Here's how the part is built. I have some questions about the finished solid (model axes, mm). A direction names the side the tool comes from. Round coordinates to 2 decimals unless told otherwise and drop trailing zeros. Loops run counter-clockwise (first coordinate to the right, second up) from the corner with the lowest first, then second, coordinate; pieces in that order, holes last. Notation, with made-up numbers: (63, 84) - (92, 84) arc R22 cw to (92, 101) - close; hole circle Ø4 at (-20, 36). An arc over 180 degrees is marked (long way). Answer as a JSON object with one key per item and string values. Group by question number.
1) I want a section at B-B, the plane z = 1.75. Give the number of separate pieces and of enclosed holes in the cut face, then the cut area to 3 significant figures.
2) I want a section at A-A, the plane y = 2. Please give me the cut outline in (x, z).
3) If we mould it in two halves opening along X, with no side actions, what happens to faces 1 (the face through (29.626, 11.272, 3.904)), 2 (the face through (6.35, 12.19, 2.4))? For each: pulls with the +X half, pulls with the -X half, needs draft (parallel to the pull), parting line crosses it, or undercut.
4) If I drill on line 1 along X through (y, z) = (25.4, 2.25); line 2 along X through (y, z) = (13, 2.05); line 3 along Y through (x, z) = (24.8, 2.7), over which ranges is the centre line in solid material (lowest first)? Write a range as [from, to].
5) I want a section at C-C, the plane x = 9. Please give me the cut outline in (y, z), then the cut area to 3 significant figures.
6) Will these pins go through, and if not, where does the flat tip stop? P1, Ø6, axis at x = 12.5, y = 11.5, coming from the +Z side; P2, Ø0.5, axis at y = 17, z = 4, coming from the +X side; P3, Ø1.4, axis at x = 6.6, y = 20.8, coming from the +Z side.
7) Which directions (+Z, -Z, +X, -X, +Y, -Y) give clear straight access to the entire face, cutting with the end or side of a thin tool? Please do faces 3 (the face through (14.657, 1.622, 5.502)), 4 (the face through (28.2, 24.2, 6.6)), 5 (the face through (15, 0, 4)), 6 (the face through (29.778, 18.074, 5.038)).
8) I want a section at D-D, the plane y = 14.25. Please give me the cut outline in (x, z), then the cut area to 3 significant figures.
Autodesk Inventor part; units mm, degrees
ref_plane "YZ Plane" through (0, 0, 0) normal (1, 0, 0) x (0, 1, 0)
ref_plane "XZ Plane" through (0, 0, 0) normal (0, 1, 0) x (-1, 0, 0)
ref_plane "XY Plane" through (0, 0, 0) normal (0, 0, 1) x (1, 0, 0)
sketch "Sketch1" plane through (0, 0, 0) normal (0, 0, 1) x (1, 0, 0)
  line L0 (0, 0) -> (31.4, 0)
  line L1 (31.4, 0) -> (31.4, 27.4)
  line L2 (31.4, 27.4) -> (0, 27.4)
  line L3 (0, 27.4) -> (0, 0)
  dimension "d0" = 31.4
  dimension "d1" = 27.4
extrude "Extrusion1" add sketch "Sketch1" along normal blind 4.17
sketch "Sketch2" plane through (0, 0, 4.17) normal (0, 0, 1) x (1, 0, 0)
  line L0 (0, 0) -> (0, 27.4)
  line L1 (31.4, 0) -> (0, 0)
  line L2 (31.4, 27.4) -> (31.4, 0)
  line L3 (0, 27.4) -> (31.4, 27.4)
  line L4 (3.2, 3.2) -> (28.2, 3.2)
  line L5 (28.2, 3.2) -> (28.2, 24.2)
  line L6 (28.2, 24.2) -> (3.2, 24.2)
  line L7 (3.2, 24.2) -> (3.2, 3.2)
  line L8 (3.2, 24.2) -> (4.6142, 22.7858)
  line L9 (28.2, 24.2) -> (26.7858, 22.7858)
  line L10 (28.2, 3.2) -> (26.7858, 4.6142)
  line L11 (3.2, 3.2) -> (4.6142, 4.6142)
  circle A0 centre (4.6142, 22.7858) radius 2
  circle A1 centre (26.7858, 22.7858) radius 2
  circle A2 centre (26.7858, 4.6142) radius 2
  circle A3 centre (4.6142, 4.6142) radius 2
  dimension "d11" = 4
  dimension "d12" = 4
  dimension "d13" = 4
  dimension "d14" = 4
  dimension "d4" = 3.2
  dimension "d5" = 3.2
  dimension "d6" = 3.2
  dimension "d8" = 3.2
  dimension "d9" = 45
  dimension "d10" = 45
extrude "Extrusion2" add sketch "Sketch2" along normal blind 4.83
sketch "Sketch3" plane through (0, 0, 9) normal (0, 0, 1) x (1, 0, 0)
  line L0 (0, 27.4) -> (31.4, 27.4)
  line L1 (0, 0) -> (0, 27.4)
  line L2 (31.4, 0) -> (0, 0)
  line L3 (31.4, 27.4) -> (31.4, 0)
  point P0 (2, 25.4)
  point P1 (29.4, 25.4)
  point P2 (29.4, 2)
  point P3 (2, 2)
  dimension "d17" = 2
  dimension "d18" = 2
  dimension "d19" = 2
  dimension "d20" = 2
  dimension "d21" = 2
  dimension "d22" = 2
  dimension "d23" = 2
  dimension "d24" = 2
hole "Hole1" at (2, 25.4, 9) at (29.4, 25.4, 9) at (29.4, 2, 9) at (2, 2, 9) direction (0, 0, -1) diameter 1.6942 end through all
sketch "Sketch6" plane through (31.4, 0, 0) normal (1, 0, 0) x (0, 0, -1)
  line L0 (0, 0) -> (0, 27.4)
  line L1 (0, 27.4) -> (-9, 27.4)
  point P0 (-4.8, 17)
  dimension "d50" = 4.8
  dimension "d51" = 10.4
hole "Hole4" at (31.4, 17, 4.8) direction (-1, 0, 0) diameter 2.2 depth 3.2
sketch "Sketch7" plane through (31.4, 0, 0) normal (1, 0, 0) x (0, 0, -1)
  circle A0 centre (-4.8, 17) radius 1.1
  point P0 (-4.8, 23.1)
  point P1 (-4.8, 10.9)
  dimension "d59" = 6.1
  dimension "d60" = 6.1
hole "Hole5" at (31.4, 23.1, 4.8) at (31.4, 10.9, 4.8) direction (-1, 0, 0) diameter 1.9406 depth 3.5 tip angle 118
sketch "Sketch10" plane through (0, 0, 4.17) normal (0, 0, 1) x (1, 0, 0)
  line L0 (0, 27.4) -> (31.4, 27.4)
  line L1 (6.6, 20.8) -> (24.8, 20.8) construction
  line L2 (24.8, 20.8) -> (24.8, 13) construction
  line L3 (24.8, 13) -> (6.6, 13) construction
  line L4 (6.6, 13) -> (6.6, 20.8) construction
  line L5 (0, 0) -> (0, 27.4) construction
  dimension "d170" = 6.6
  dimension "d171" = 6.6
  dimension "d172" = 7.8
  dimension "d173" = 18.2
hole "Hole8" at (6.6, 20.8, 4.17) at (6.6, 13, 4.17) at (24.8, 13, 4.17) at (24.8, 20.8, 4.17) direction (0, 0, -1) diameter 1.6942 depth 3.5 tip angle 118
sketch "Sketch15" plane through (0, 0, 0) normal (0, -1, 0) x (1, 0, 0)
  line L0 (0, 0) -> (0, 9) construction
  line L1 (0, 6) -> (31.3856, 6) construction
  line L2 (0, 0) -> (31.4, 0) construction
  line L3 (31.4, 9) -> (0, 9) construction
  line L4 (5.7, 9) -> (5.7, 0) construction
  point P0 (9.7, 6)
  point P1 (13.7, 6)
  point P2 (5.7, 6)
  dimension "d133" = 6
  dimension "d136" = 5.7
  dimension "d137" = 4
  dimension "d138" = 8
hole "Hole13" at (9.7, 0, 6) at (13.7, 0, 6) direction (0, 1, 0) diameter 2.1565 depth 3.2 tip angle 118
hole "Hole15" at (5.7, 0, 6) direction (0, 1, 0) diameter 1.6942 depth 3.2 tip angle 118
equation "\"d12\" = d11"
equation "\"d13\" = d11"
equation "\"d14\" = d11"
equation "\"d5\" = d4"
equation "\"d6\" = d4"
equation "\"d8\" = d4"
equation "\"d10\" = d9"
properties part number "Mixer IQ Box ND20" material "Aluminum-6061"
Outcome:
{
 "1": {"separate pieces": "1", "enclosed holes": "8", "area": "842 mm^2"},
 "2": {"outline": "(0, 0) - (1.15, 0) - (1.15, 9) - (0, 9) - close; (2.85, 0) - (28.55, 0) - (28.55, 9) - (2.85, 9) - close; (30.25, 0) - (31.4, 0) - (31.4, 9) - (30.25, 9) - close; hole circle Ø1.69 at (5.7, 6); hole circle Ø2.16 at (9.7, 6); hole circle Ø2.16 at (13.7, 6)"},
 "3": {"face 1": "needs draft", "face 2": "undercut"},
 "4": {"line 1": "[0, 1.15], [2.85, 28.55], [30.25, 31.4]", "line 2": "[0, 5.75], [7.45, 23.95], [25.65, 31.4]", "line 3": "[0, 12.15], [13.85, 19.95], [21.65, 27.4]"},
 "5": {"outline": "(0, 0) - (27.4, 0) - (27.4, 9) - (24.2, 9) - (24.2, 4.17) - (3.2, 4.17) - (3.2, 5.18) - (0, 5.18) - close; (0, 6.82) - (3.2, 6.82) - (3.2, 9) - (0, 9) - close", "area": "140 mm^2"},
 "6": {"P1": "z = 4.17", "P2": "x = 28.2", "P3": "z = 0.58"},
 "7": {"face 3": "-Y", "face 4": "+Z", "face 5": "+Z, -Z, +X, -X, -Y", "face 6": "+X"},
 "8": {"outline": "(0, 0) - (31.4, 0) - (31.4, 9) - (28.2, 9) - (28.2, 4.17) - (3.2, 4.17) - (3.2, 9) - (0, 9) - close", "area": "162 mm^2"}
}
